Geometry: see drawing. Coordinates: mm, zero at the bounding-box minimum. Give positions to 0.01 mm unless a question says otherwise; leave off trailing zeros. Write each loop counter-clockwise with the first axis right and the second up, starting at its lowest first coordinate (ties: lowest second). Pieces come first, ordered by that corner, then holes. Notation, with made-up numbers: M -16.5,80.5 L 9.5,80.5 A22 ccw 9.5,110.5 Z; hole C 45,-2 d7. An arc over 180 degrees is marked long. Use a Markdown table: item, result. Add a question column.
1) Line query: line 1 (X direction, y = 1.65, z = 41); line 2 (X direction, y = 0.85, z = 22). Output: solid intervals per line, ascending.
2) Section A-A on x = 3. Return the cut outline in (y, z).
3) Section C-C on y = 1.1. Return the cut outline in (x, z), then the cut area to 3 significant figures.
4) Section B-B on z = 41. Return the cut outline in (x, y), then the cut area to 3 significant figures.
5) Section D-D on x = 32. Return the cut outline in (y, z), then the cut area to 3 significant figures.
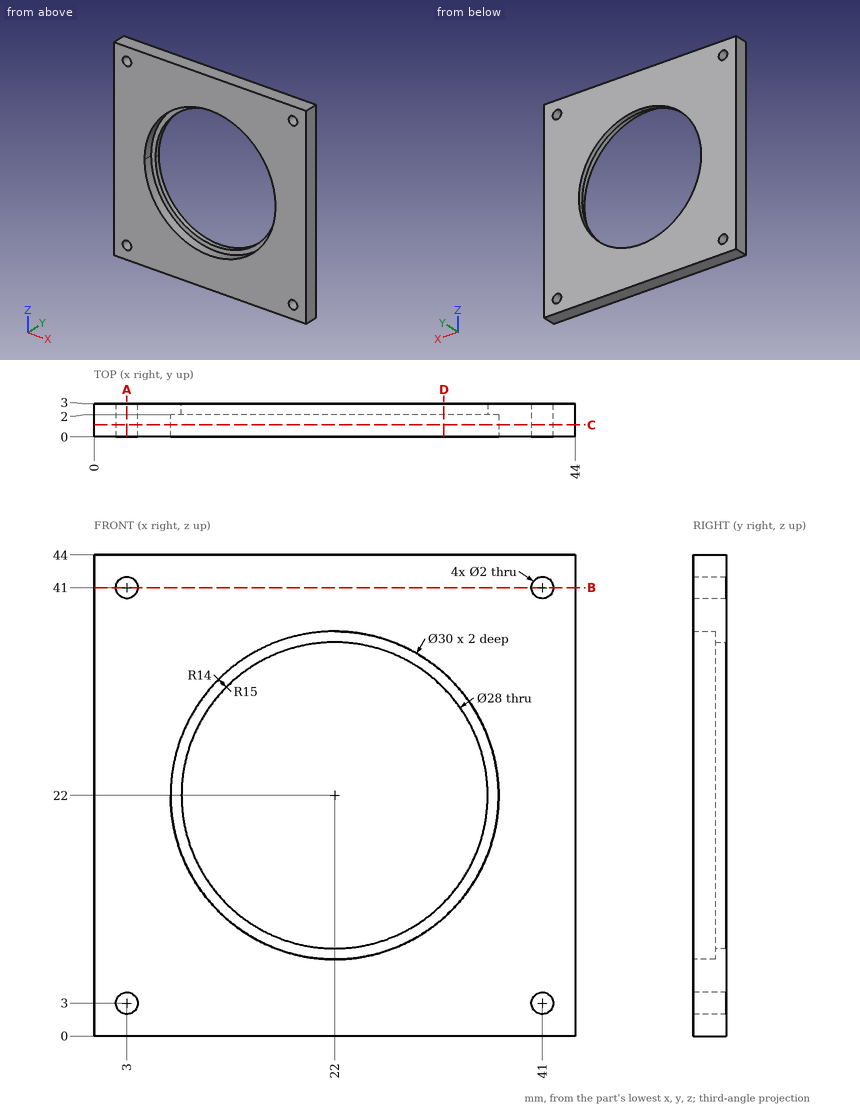
Found:
| question | item | result |
|---|---|---|
| 1 | line 1 | 0 to 2, 4 to 40, 42 to 44 |
| 1 | line 2 | 0 to 7, 37 to 44 |
| 2 | outline | M 0,0 L 3,0 L 3,2 L 0,2 Z; M 0,4 L 3,4 L 3,40 L 0,40 Z; M 0,42 L 3,42 L 3,44 L 0,44 Z |
| 3 | outline | M 0,0 L 44,0 L 44,44 L 0,44 Z; hole C 3,3 d2; hole C 3,41 d2; hole C 22,22 d30; hole C 41,3 d2; hole C 41,41 d2 |
| 3 | area | 1,220 mm² |
| 4 | outline | M 0,0 L 2,0 L 2,3 L 0,3 Z; M 4,0 L 40,0 L 40,3 L 4,3 Z; M 42,0 L 44,0 L 44,3 L 42,3 Z |
| 4 | area | 120 mm² |
| 5 | outline | M 0,0 L 3,0 L 3,12.2 L 2,12.2 L 2,10.82 L 0,10.82 Z; M 0,33.18 L 2,33.18 L 2,31.8 L 3,31.8 L 3,44 L 0,44 Z |
| 5 | area | 67.7 mm² |
